from build123d import *

# Parameters (mm, degrees)
BOSS_EXTRUDE1_DEPTH     = 9
CHAMFER1_SIZE           = 1
SKETCH2_R               = 3
CUT_EXTRUDE2_DEPTH      = 27.5
CUT_EXTRUDE2_DEPTH_BACK = 27.5
SKETCH2_3_R             = 3
SKETCH2_3_R_2           = 2
BOSS_EXTRUDE2_DEPTH     = 7
SKETCH3_W               = 1.5
SKETCH3_H               = 7.004177156
CUT_EXTRUDE3_DEPTH      = 1
CUT_EXTRUDE3_DEPTH_BACK = 10


with BuildPart() as part:
    # Sketch1 → Boss-Extrude1 (new body)
    with BuildSketch(Plane(origin=(0, 0, 0), x_dir=(1, 0, 0), z_dir=(0, 1, 0))):
        with BuildLine():
            Line((-0.75, 21), (0.75, 21))
            Line((0.75, 21), (0.75, 17.483921185))
            ThreePointArc((0.75, 17.483921185), (17.5, 0), (0.75, -17.483921185))
            Line((0.75, -17.483921185), (0.75, -26.489384666))
            ThreePointArc((0.75, -26.489384666), (0, 26.5), (-0.75, -26.489384666))
            Line((-0.75, -26.489384666), (-0.75, -17.483921185))
            ThreePointArc((-0.75, -17.483921185), (-17.5, 0), (-0.75, 17.483921185))
            Line((-0.75, 17.483921185), (-0.75, 21))
        make_face()
    extrude(amount=BOSS_EXTRUDE1_DEPTH)

    # Chamfer1
    chamfer1_edges = [part.edges().sort_by_distance(p)[0] for p in [
        (-17.5, 0, 0),
        (0, 0, -26.5),
        (-17.5, 9, 0),
        (17.5, 9, 0),
        (0, 9, -26.5),
        (17.5, 0, 0),
    ]]
    chamfer(chamfer1_edges, length=CHAMFER1_SIZE)

    # Sketch2 → Cut-Extrude2 (cut, two sides)
    with BuildSketch(Plane(origin=(0, 0, 0), x_dir=(0, 0, -1), z_dir=(1, 0, 0))) as cut_extrude2_sk:
        with Locations((-22, 4.5)):
            Circle(SKETCH2_R)
    extrude(amount=CUT_EXTRUDE2_DEPTH, mode=Mode.SUBTRACT)
    extrude(cut_extrude2_sk.sketch, amount=-CUT_EXTRUDE2_DEPTH_BACK, mode=Mode.SUBTRACT)

    # Sketch2<3> → Boss-Extrude2 (add, symmetric)
    with BuildSketch(Plane(origin=(0, 0, 0), x_dir=(0, 0, -1), z_dir=(1, 0, 0))):
        with Locations((-22, 4.5)):
            Circle(SKETCH2_3_R)
        with Locations((-22, 4.5)):
            Circle(SKETCH2_3_R_2, mode=Mode.SUBTRACT)
    extrude(amount=BOSS_EXTRUDE2_DEPTH, both=True)

    # Sketch3 → Cut-Extrude3 (cut, two sides)
    with BuildSketch(Plane(origin=(0, 9, 0), x_dir=(1, 0, 0), z_dir=(0, 1, 0))) as cut_extrude3_sk:
        with Locations((0, -21.986879624)):
            Rectangle(SKETCH3_W, SKETCH3_H)
    extrude(amount=CUT_EXTRUDE3_DEPTH, mode=Mode.SUBTRACT)
    extrude(cut_extrude3_sk.sketch, amount=-CUT_EXTRUDE3_DEPTH_BACK, mode=Mode.SUBTRACT)


solid = part.part
The listing builds one solid part. Answer for the finished solid, in the listing's coordinates (mm). A direction names the side the tool comes from. Round coordinates to 2 decimals unless told otherwise and drop trailing zeros. Write each loop counter-clockwise with the first axis right and the second up, starting at its lowest first coordinate (ties: lowest second). Pieces come first, ordered by that corner, then holes. Notation, with made-up numbers: M 75.5,72 L 94.5,72 A25 ccw 94.5,92 Z; hole C 17.25,-15 d6. An arc over 180 degrees is marked long. Write each question's results on one line, items separated by ' | '. Start each with the question number.
Item 1: Find section B-B on x = 0. Write down the section's boundary in (y, z).
Item 2: The mould has two halves that part along X. Classify faces 1 (the flat face through (7, 7, 22)), 2 (the flat face through (-13.3, 0, 13.1)), 3 (the flat face through (0, 4, -21)): +X half, -X half, draft (parallel to the pull), parting line (faces both ways), or undercut.
Item 3: Straight lines are drawn through the part: probe 1 along Y at (x, z) = (-2, 22); probe 2 along X at (y, z) = (2, 22.5); probe 3 along Y at (x, z) = (-12, 22). For each, find the intervals that lie inside material, in ascending order.
Item 4: Which of the six approach directions +Z, -Z, +X, -X, +Y, -Y give full straight-line access (tool end or side, diameter ignored) to faces 4 (the conical face through (-17.67, 0.826, 0.379)), 5 (the flat face through (-0.75, 2, 22)), 6 (the cylindrical face through (-11.38, 5.4, 19.14))?
Item 5: Given pin 1 Ø2 at (y, z) = (7, -14.5) entering from -X; pin 2 Ø3 at (x, y) = (-15, 1.5) entering from +Z; pin 3 Ø4.5 at (y, z) = (4.5, 21) entering from +X; pin 4 Ø3.5 at (y, z) = (4.5, 22) entering from -X, each flat-ended and moving along its own axis, determine where each tip first touches the part or whether it passes through.
Item 6: Find section C-C on z = 22. Give the number of separate pieces and of enclosed holes in the cut face, and give its area (3 significant figures).
Item 7: Find section A-A on z = 0. Write down the section's boundary in (x, y), and give its area (3 significant figures).
Answer block:
1) outline: M 0,-25.5 L 1,-26.5 L 8,-26.5 L 9,-25.5 L 9,-21 L 0,-21 Z
2) face 1: +X half | face 2: draft | face 3: undercut
3) probe 1: y = 0 to 2.5, 6.5 to 9 | probe 2: x = -7 to -0.75, 0.75 to 7 | probe 3: y = 0 to 1.5, 7.5 to 9
4) face 4: -Y | face 5: +Z, +Y, -Y | face 6: -X
5) pin 1: stops at x = -22.8 | pin 2: stops at z = 22.8 | pin 3: stops at x = 18.73 | pin 4: passes through
6) separate pieces: 4 | enclosed holes: 0 | area: 105 mm²
7) outline: M -26.5,1 L -25.5,0 L -18.5,0 L -17.5,1 L -17.5,8 L -18.5,9 L -25.5,9 L -26.5,8 Z; M 17.5,1 L 18.5,0 L 25.5,0 L 26.5,1 L 26.5,8 L 25.5,9 L 18.5,9 L 17.5,8 Z | area: 158 mm²
